Design review of the part built by this model. Coordinates are the model's own, in mm. Round coordinates to 2 decimals unless told otherwise and drop trailing zeros. Write each loop counter-clockwise with the first axis right and the second up, starting at its lowest first coordinate (ties: lowest second). Pieces come first, ordered by that corner, then holes. Notation, with made-up numbers: (25, 35.5) -> (71, 35.5) arc R32 cw to (71, 72.5) -> close; hole circle Ø9 at (69.25, -6.75). An arc over 180 degrees is marked (long way). Write item = value, one per line. Start each with the question number.
Item 1: Add section A-A, the plane x = -32. State the section outline as (y, z) points, then the cut area to 3 significant figures.
Item 2: To check wall thickness, follow L1, parallel to Y at x = 0, z = 0.1; L2, parallel to X at y = 15, z = 0.15; L3, parallel to X at y = -13.5, z = 0.1. State the ranges of each line that lie inside material, in increasing order.
Item 3: Add section C-C, the plane z = 0.15. State the section outline as (x, y) points, then the cut area to 3 significant figures.
Item 4: Add section B-B, the plane y = 0. State the section outline as (x, z) points, then the cut area to 3 significant figures.
Autodesk Inventor part; units mm, degrees
ref_plane "YZ Plane" through (0, 0, 0) normal (1, 0, 0) x (0, 1, 0)
ref_plane "XZ Plane" through (0, 0, 0) normal (0, 1, 0) x (-1, 0, 0)
ref_plane "XY Plane" through (0, 0, 0) normal (0, 0, 1) x (1, 0, 0)
sketch "Sketch1" plane through (0, 0, 0) normal (0, 0, 1) x (1, 0, 0)
  line L0 (-35, 35) -> (35, 35)
  line L1 (35, 35) -> (35, -35)
  line L2 (35, -35) -> (-35, -35)
  line L3 (-35, -35) -> (-35, 35)
  circle A0 centre (0, 0) radius 30
  point P0 (35, 0)
  point P1 (0, 35)
  dimension "d0" = 70
  dimension "d1" = 60
extrude "Extrusion1" add sketch "Sketch1" along normal blind 0.2
chamfer "Chamfer1" distance 12 angle 45 4 edges at (35, 35, 0.1) (35, -35, 0.1) (-35, -35, 0.1) (-35, 35, 0.1)
fillet "Fillet1" radius 2 8 edges at (-23, 35, 0.1) (23, 35, 0.1) (35, 23, 0.1) (35, -23, 0.1) (23, -35, 0.1) (-23, -35, 0.1) (-35, -23, 0.1) (-35, 23, 0.1)
sketch "Sketch2" plane through (0, 0, 0.2) normal (0, 0, 1) x (1, 0, 0)
  circle A0 centre (0, 0) radius 32 construction
  point P0 (32, 0)
  dimension "d8" = 64
hole "Hole1" at (32, 0, 0.2) direction (0, 0, -1) diameter 3.2 end through all
pattern_circular "Circular Pattern1" count 4 over 360 about axis through (0, 0, -10) along (0, 0, 1) of "Hole1"
sketch "Sketch3" plane through (0, 0, 0.2) normal (0, 0, 1) x (1, 0, 0)
  circle A0 centre (0, 0) radius 23.75 construction
  point P0 (23.75, 0)
  dimension "d19" = 47.5
properties part number "plasma-box-mica" material "Nylon 6/6"
Result set:
q1.outline = (-26, 0) -> (-1.6, 0) -> (-1.6, 0.2) -> (-26, 0.2) -> close; (1.6, 0) -> (26, 0) -> (26, 0.2) -> (1.6, 0.2) -> close
q1.area = 9.76 mm²
q2.L1 = -35 to -33.6, -30.4 to -30, 30 to 30.4, 33.6 to 35
q2.L2 = -35 to -25.98, 25.98 to 35
q2.L3 = -35 to -26.79, 26.79 to 35
q3.outline = (-35, -22.17) arc R2 ccw to (-34.41, -23.59) -> (-23.59, -34.41) arc R2 ccw to (-22.17, -35) -> (22.17, -35) arc R2 ccw to (23.59, -34.41) -> (34.41, -23.59) arc R2 ccw to (35, -22.17) -> (35, 22.17) arc R2 ccw to (34.41, 23.59) -> (23.59, 34.41) arc R2 ccw to (22.17, 35) -> (-22.17, 35) arc R2 ccw to (-23.59, 34.41) -> (-34.41, 23.59) arc R2 ccw to (-35, 22.17) -> close; hole circle Ø3.2 at (-32, 0); hole circle Ø60 at (0, 0); hole circle Ø3.2 at (0, -32); hole circle Ø3.2 at (0, 32); hole circle Ø3.2 at (32, 0)
q3.area = 1,750 mm²
q4.outline = (-35, 0) -> (-33.6, 0) -> (-33.6, 0.2) -> (-35, 0.2) -> close; (-30.4, 0) -> (-30, 0) -> (-30, 0.2) -> (-30.4, 0.2) -> close; (30, 0) -> (30.4, 0) -> (30.4, 0.2) -> (30, 0.2) -> close; (33.6, 0) -> (35, 0) -> (35, 0.2) -> (33.6, 0.2) -> close
q4.area = 0.720 mm²
